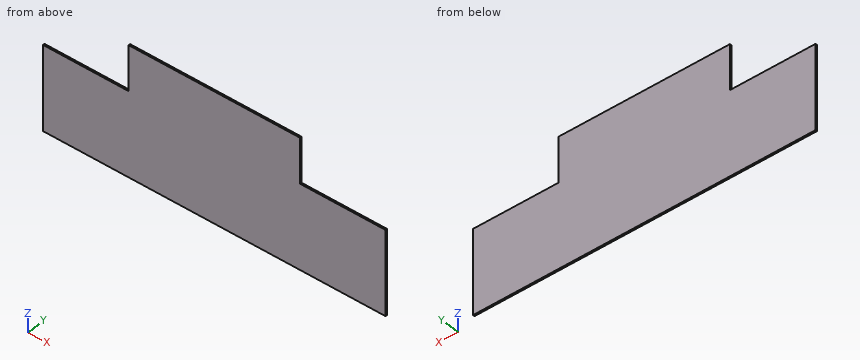
```python
from build123d import *

# Parameters (mm, degrees)
F0_W     = 600
F0_H     = 230
F1_DEPTH = 3
F2_W     = 150
F2_H     = 80
F3_DEPTH = 3.001
F4_W     = 150
F4_H     = 80
F5_DEPTH = 3.001


with BuildPart() as f1:
    # F0 (on Front) → F1 (new body)
    with BuildSketch(Plane.XZ):
        Rectangle(F0_W, F0_H)
    extrude(amount=F1_DEPTH)

    # F2 (on face) → F3 (cut, through all)
    with BuildSketch(Plane.XZ.offset(3)):
        with Locations((-225, 75)):
            Rectangle(F2_W, F2_H)
    extrude(amount=-F3_DEPTH, mode=Mode.SUBTRACT)

    # F4 (on face) → F5 (cut, through all)
    with BuildSketch(Plane.XZ.offset(3)):
        with Locations((225, 75)):
            Rectangle(F4_W, F4_H)
    extrude(amount=-F5_DEPTH, mode=Mode.SUBTRACT)


solid = f1.part
```
Could you check a few things on this model? Use its own coordinates, in mm. Round coordinates to 2 decimals unless told otherwise and drop trailing zeros. Loops run counter-clockwise (first coordinate to the right, second up) from the corner with the lowest first, then second, coordinate; pieces in that order, holes last. Notation, with made-up numbers: M 8.25,20 L 20.25,20 A22 ccw 20.25,49 Z; hole C -13,-4 d10. An arc over 180 degrees is marked long. Put each result on its own line as item: value.
Q1. For pin 1 (1.5 mm diameter, centred on x = 202.5, y = -1, fed in from +Z); pin 2 (12 mm diameter, centred on x = 175, z = -54.5, fed in from +Y); pin 3 (0.9 mm diameter, centred on y = -1.5, z = 59.5, fed in from +X), each with a flat end and sliding along its axis, tell me the tip position at first contact or that it passes through.
Check result:
pin 1: z = 35
pin 2: y = 0
pin 3: x = 150
Q2. Imagine slicing it at A-A (y = -1.4). Write out the boundary of the cut face in (x, z).
Check result:
outline: M -300,-115 L 300,-115 L 300,35 L 150,35 L 150,115 L -150,115 L -150,35 L -300,35 Z
Q3. Imagine slicing it at B-B (z = 88.5). Write out the boundary of the cut face in (x, y), then the cut area to 3 significant figures.
Check result:
outline: M -150,-3 L 150,-3 L 150,0 L -150,0 Z
area: 900 mm2
Q4. Imagine slicing it at C-C (x = 176.5). Write out the boundary of the cut face in (y, z).
Check result:
outline: M -3,-115 L 0,-115 L 0,35 L -3,35 Z
Q5. I need wall thicknesses on probe 1 along X at (y, z) = (-2.9, 42); probe 2 along Z at (x, y) = (223.5, -2.25). Which ranges of each line are inside material? Lowest first, please.
Check result:
probe 1: -150 to 150
probe 2: -115 to 35
